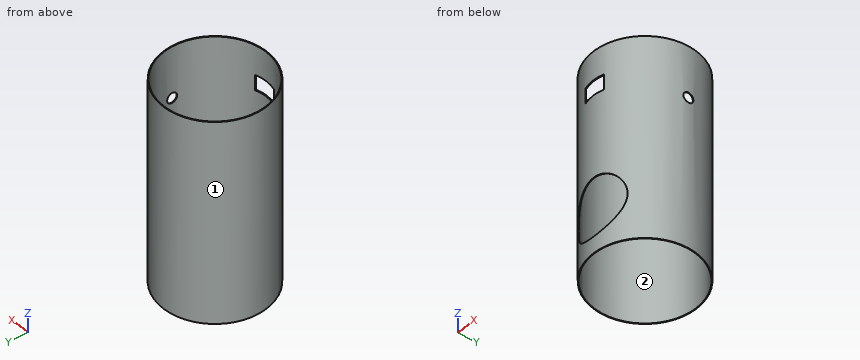
Autodesk Inventor part; units mm, degrees
ref_plane "WeldJoint" through (0, 0, -10) normal (0.5, -0.866, 0) x (0, 0, 1)
ref_plane "Inlet_Clock_Angle_plane" through (0, 0, -10) normal (0, 1, 0) x (0, 0, 1)
ref_plane "Charging" through (0, 0, -10) normal (1, 0, 0) x (0, 0, 1)
sketch "Sketch13" plane through (0, 0, 0) normal (0, 0, 1) x (1, 0, 0)
  circle A0 centre (0, 0) radius 470 construction
  line L0 (0, 0) -> (0, -470)
  line L1 (0, 0) -> (-407.0319, -235)
  line L2 (0, 0) -> (470, 0)
  line L3 (0, 0) -> (0, -470)
  line L4 (0, 0) -> (0, -470)
  line L5 (0, 0) -> (418.7731, 213.3755)
  line L6 (0, 0) -> (0, 470)
  dimension "d53" = 940
  dimension "d55" = 0
  dimension "d98" = 180
  dimension "d99" = 240
  dimension "d100" = 63
  dimension "d101" = 90
ref_plane "WeldJoint" through (0, 0, -10) normal (0.5, -0.866, 0) x (0, 0, 1)
ref_plane "Inlet_Clock_Angle_plane" through (0, 0, -10) normal (0, 1, 0) x (0, 0, 1)
ref_plane "Charging" through (0, 0, -10) normal (1, 0, 0) x (0, 0, 1)
ref_plane "Accsess" through (0, 0, -10) normal (1, 0, 0) x (0, 0, 1)
sketch "Sketch14" plane through (0, 0, -10) normal (0.5, -0.866, 0) x (0, 0, 1)
  line L0 (1842, 464) -> (10, 464)
  line L1 (10, 464) -> (10, 470)
  line L2 (10, 470) -> (1842, 470)
  line L3 (1842, 470) -> (1842, 464)
  line L4 (10, 0) -> (1842, 0)
  line L5 (10, 470) -> (-20, 470) construction
  line L6 (10, 464) -> (-20, 464) construction
  arc A0 (-20, 464) -> (-74.1579, 429.8249) centre (-20, 404) ccw construction
  arc A1 (-74.1579, 429.8249) -> (-168, 15) centre (795.7784, 15) ccw construction
  line L7 (-168, 15) -> (-168, 0) construction
  line L8 (10, 0) -> (-168, 0) construction
  arc A2 (-20, 470) -> (-79.5736, 432.4074) centre (-20, 404) ccw construction
  arc A3 (-79.5736, 432.4074) -> (-174, 15) centre (795.7784, 15) ccw construction
  line L9 (-174, 15) -> (-174, 0) construction
  line L10 (-168, 0) -> (-174, 0) construction
  line L11 (1842, 464) -> (1872, 464)
  line L12 (1842, 470) -> (1872, 470)
  line L13 (1842, 0) -> (2020, 0) construction
  line L14 (2026, 0) -> (2026, 15) construction
  arc A4 (2026, 15) -> (1931.5736, 432.4074) centre (1056.2216, 15) ccw construction
  arc A5 (1931.5736, 432.4074) -> (1872, 470) centre (1872, 404) ccw construction
  line L15 (2020, 0) -> (2020, 15) construction
  line L16 (2020, 0) -> (2026, 0) construction
  arc A6 (2020, 15) -> (1926.1579, 429.8249) centre (1056.2216, 15) ccw construction
  arc A7 (1926.1579, 429.8249) -> (1872, 464) centre (1872, 404) ccw construction
  line L17 (-119.3891, 418.399) -> (-474, 418.399)
  line L18 (-474, 418.399) -> (-474, 338.399)
  line L19 (-474, 338.399) -> (-119.3891, 338.399)
  line L20 (-119.3891, 338.399) -> (-119.3891, 418.399)
  line L21 (2026, 15) -> (2056, 15) construction
  line L22 (2056, 15) -> (2056, 0) construction
  line L23 (2056, 0) -> (2026, 0) construction
  line L24 (-474, 498.399) -> (-474, 418.399)
  line L25 (-474, 498.399) -> (-468, 498.399)
  line L26 (-468, 498.399) -> (-468, 418.399)
  line L27 (-81.71, 432.3205) -> (-126.8357, 319.837)
  line L28 (-119.3891, 418.399) -> (-87.295, 418.399)
  line L29 (-74.1579, 429.8249) -> (-79.5736, 432.4074)
  line L30 (-81.71, 432.3205) -> (-81.3377, 433.2486) construction
  line L31 (-81.3377, 433.2486) -> (-79.5736, 432.4074) construction
  line L32 (-474, 498.399) -> (-474, 498.399)
  line L33 (-474, 498.399) -> (-474, 338.399)
  line L34 (-474, 338.399) -> (-474, 338.399)
  line L35 (1421, 470) -> (1331, 470)
  line L36 (1331, 470) -> (1331, 570)
  line L37 (1331, 570) -> (1421, 570)
  line L38 (1421, 570) -> (1421, 470)
  point P0 (10, 467)
  point P1 (-104.2729, 376.0787)
  point P2 (1376, 570)
  dimension "d59" = 1832
  dimension "d60" = 6
  dimension "d61" = 940
  dimension "d82" = 60
  dimension "d83" = 30
  dimension "d86" = 80
  dimension "d87" = 30
  dimension "d91" = 15
  dimension "d92" = 20
  dimension "d93" = 184
  dimension "d94" = 30
  dimension "d103" = 386.705
  dimension "d104" = 21.86
  dimension "d105" = 121.1976
  dimension "d107" = 1
  dimension "d108" = 676.798
  dimension "d109" = 0
  dimension "d110" = 2530
  dimension "d111" = 300
  dimension "d112" = 100
  dimension "d113" = 90
  dimension "d114" = 1850
  dimension "d115" = 1366
revolve "Revolution2" add sketch "Sketch14" angle 359.9 about axis through (0, 0, 0) along (0, 0, 1) contours L0 L1 L2 L3
sketch "Sketch AnglePlane_InletPipe" plane through (0, 0, -10) normal (0, 1, 0) x (0, 0, 1)
  line L0 (10, -470) -> (10, 470)
  line L1 (10, 0) -> (1376, 0)
  line L2 (1376, 0) -> (1376, 470)
  line L3 (1376, 470) -> (10, 470)
  line L4 (10, 470) -> (10, 0)
  point P0 (10, -407.0319)
  point P1 (10, -407.4415)
  dimension "d63" = 940
  dimension "d64" = 90
  dimension "frd_hght" = 1366
ref_plane "InletPipe_AnglePlane" through (0, 0, 1366) normal (1, 0, 0) x (0, 1, 0)
sketch "Sketch16" plane through (0, 0, 1366) normal (1, 0, 0) x (0, 1, 0)
  circle A0 centre (0, 0) radius 45.5
  point P0 (0, -1366)
  point P1 (0, 0)
  point P2 (0, 0)
  point P3 (0, 0)
  dimension "d66" = 91
extrude "Extrusion7" cut sketch "Sketch16" along normal through all
ref_plane "Work Plane16" through (0, 0, 0) normal (0, -1, 0) x (1, 0, 0)
sketch "Sketch17" plane through (0, 0, 0) normal (0, -1, 0) x (1, 0, 0)
  circle A0 centre (0, 417.5) radius 267.5
  line L0 (0, 150) -> (-495.5727, 150)
  point P0 (0, 0)
  dimension "d69" = 535
  dimension "d71" = 150
extrude "Extrusion8" cut sketch "Sketch17" along normal through all
sketch "ChargingAngleSketch19" plane through (0, 0, -10) normal (1, 0, 0) x (0, 0, 1)
  line L0 (10, 0) -> (1170.6454, 0)
  line L1 (1170.6454, 0) -> (1442, 470)
  line L2 (1442, 470) -> (10, 470)
  line L3 (10, 470) -> (10, 0)
  dimension "d74" = 1432
  dimension "d76" = 940
  dimension "d77" = 60
ref_plane "Work Plane18" through (0, 0, 1160.6454) normal (0, -0.866, 0.5) x (1, 0, 0)
sketch "Sketch20" plane through (0, 0, 1160.6454) normal (0, -0.866, 0.5) x (1, 0, 0)
  line L0 (-100, 0) -> (100, 0)
  line L1 (100, 0) -> (100, 120)
  line L2 (100, 120) -> (-100, 120)
  line L3 (-100, 120) -> (-100, 0)
  point P0 (0, -1005.1484)
  point P1 (0, 0)
  point P2 (0, 0)
  point P3 (0, 0)
  point P4 (0, 0)
  dimension "d78" = 200
  dimension "d79" = 120
extrude "Charging hole" cut sketch "Sketch20" along normal through all
equation "\"BendRadius\" = Thickness"
equation "\"BendReliefWidth\" = Thickness"
equation "\"BendReliefDepth\" = 0.5 * Thickness"
equation "\"CornerReliefSize\" = 4 * Thickness"
equation "\"MinimumRemnant\" = 2 * Thickness"
equation "\"TransitionRadius\" = BendRadius"
equation "\"JacobiRadiusSize\" = BendRadius"
equation "\"GapSize\" = Thickness"
equation "\"InletPipe_horisont_angle\" = 0"
equation "\"AccsessHatch_ClockAngle\" = 0"
equation "\"ChargingHatch_ClockAgnle\" = 180deg"
equation "\"InletPipe_Clock_angle\" = 90deg"
equation "\"OutletPipe_ClockAngle\" = 63deg"
equation "\"WeldJoint_ClockAgnle\" = 240deg"
equation "\"AA_MAIN_Shell_hight\" = 1832"
equation "\"Legs_Tube_lenght\" = 386.70499"
equation "\"Legs_Upper_plate_lenght\" = 121.19761"
equation "\"Legs_Inner_diam\" = 676.79799"
equation "\"AA_MAIN_dish_hight\" = 184"
properties part number "PRS 0101 main shell D1200 940" material "Steel"
Can you work these out from the model? Positions are in its coordinate system, mm. Face numbers are marked on the shaded views. Coordinates: 2 decimals unless noted, no trailing zeros. Order: outer loops, then holes, each group sorted by start corner. A loop starts at its lowest first (then second) coordinate and runs counter-clockwise, first axis right, second up. Notation, with made-up numbers: M 60,7 L 100,7 A17 cw 100,24 Z; hole C 64.5,-30.5 d2. An arc over 180 degrees is marked long. Answer as CSV lines item,"result".
(1) I'm going to push flat-ended pins straight in: pin 1 (6 mm diameter, centred on x = -68.5, z = 313, fed in from +Y); pin 2 (5 mm diameter, centred on x = -126.5, z = 972, fed in from +Y); pin 3 (2 mm diameter, centred on x = -248.5, z = 379.5, fed in from -Y). Where does each tip first touch, or does it pass through?
Geometry check:
pin 1,"y = 465.41"
pin 2,"y = 453.35"
pin 3,"y = 391.21"
(2) Suppose I cut it at A-A on x = -130.5. Please give me the cut outline in (y, z).
Geometry check:
outline,"M -451.52,0 L -445.27,0 L -445.27,183.99 L -451.52,183.99 Z; M -451.52,651.01 L -445.27,651.01 L -445.27,1832 L -451.52,1832 Z; M 445.27,0 L 451.52,0 L 451.52,1832 L 445.27,1832 Z"
(3) If we mould it in two halves opening along Y, with no side actions, what happens to the marked faces 1 and 2? For each: released by +Y, released by -Y, zero draft, split by the parting line, or undercut.
Geometry check:
face 1,"split by the parting line"
face 2,"undercut"
(4) Please list where these lines run through material, in increasing order: L1, parallel to X at y = 0, z = 439; L2, parallel to Y at x = 335, z = 1718.
Geometry check:
L1,"-470 to -464, 464 to 470"
L2,"-329.66 to -321.05, 321.05 to 329.66"
(5) Suppose I cut it at D-D on x = 0. Please give me the cut outline in (y, z).
Geometry check:
outline,"M -470,0 L -464,0 L -464,150 L -470,150 Z; M -470,685 L -464,685 L -464,1428.54 L -470,1432 Z; M -470,1570.56 L -464,1567.1 L -464,1832 L -470,1832 Z; M 464,0 L 470,0 L 470,1832 L 464,1832 Z"
(6) Suppose I cut it at B-B on y = 254. Please give me the cut outline in (x, z).
Geometry check:
outline,"M -395.45,0 L -388.3,0 L -388.3,1832 L -395.45,1832 Z; M 388.3,0 L 395.45,0 L 395.45,1832 L 388.3,1832 Z"
(7) Suppose I cut it at C-C on z = 417.5. Please give me the cut outline in (x, y), plus the area to 3 significant figures.
Geometry check:
outline,"M -407.44,-234.29 L -402.24,-231.3 A464 cw long 267.5,-379.13 L 267.5,-386.45 A470 ccw long Z; M -407.03,-235 A470 ccw -267.5,-386.45 L -267.5,-379.13 A464 cw -401.84,-232 Z"
area,"14,200 mm^2"
